Input: dimensioned drawing with shaded views. Units: mm. Origin: part minimum x, y, z. A direction names the side the tool comes from. Coordinates: 2 decimals unless noted, no trailing zeros. Write each loop counter-clockwise with the first axis right and the second up, starting at its lowest first coordinate (ties: lowest second). Pieces come first, ordered by that corner, then holes. Notation, with made-up numbers: M 85.5,-21 L 143.5,-21 A14 cw 143.5,-8 Z; hole C 82.25,12 d2. An arc over 180 degrees is marked long. Use one line per item in the form item = value.
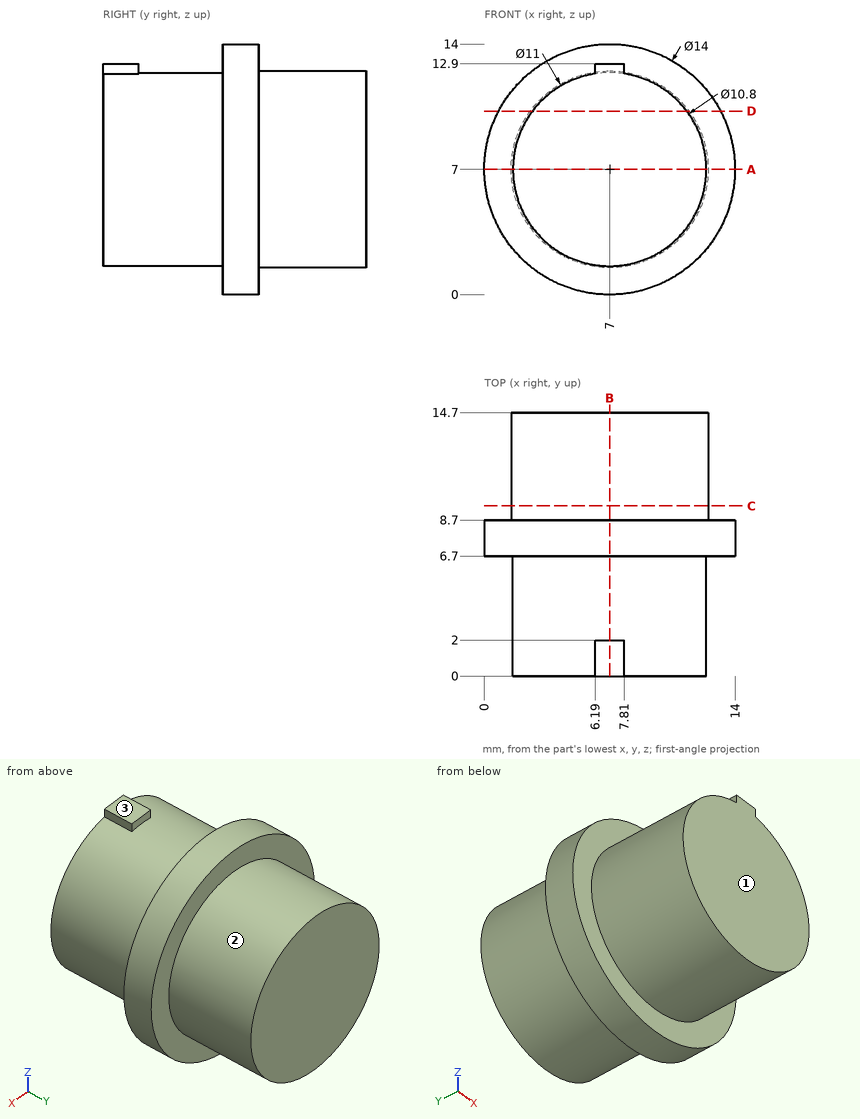
(1) Section query D-D on z = 10.25. Return the cut outline in (x, y).
Computed:
outline = M 0.8,6.7 L 2.69,6.7 L 2.69,0 L 11.31,0 L 11.31,6.7 L 13.2,6.7 L 13.2,8.7 L 11.44,8.7 L 11.44,14.7 L 2.56,14.7 L 2.56,8.7 L 0.8,8.7 Z
(2) Section query A-A on z = 7. Return the cut outline in (x, y), plus the area to 3 significant figures.
Computed:
outline = M 0,6.7 L 1.6,6.7 L 1.6,0 L 12.4,0 L 12.4,6.7 L 14,6.7 L 14,8.7 L 12.5,8.7 L 12.5,14.7 L 1.5,14.7 L 1.5,8.7 L 0,8.7 Z
area = 166 mm^2
(3) Section query C-C on y = 9.5. Return the cut outline in (x, z).
Computed:
outline = C 7,7 d11
(4) Set-up query: the marked faces 1, 2 and 3. Return all of +Z, -Z, +X, -X, +Y, -Y with unobstructed straight access to the full face (end or side cutting, diameter ignored); none if empty.
Computed:
face_1 = +Z, -Z, +X, -X, -Y
face_2 = +Y
face_3 = +Z, +X, -X, -Y
(5) First-contact query: pin 1 Ø2 at (x, z) = (3, 1.5) entering from +Y; pin 2 Ø1 at (y, z) = (6, 4.5) entering from +X; pin 3 Ø2 at (x, y) = (8, 5) entering from +Z. Flat tips, straight axial feed; report the tip coordinate or a pass-through.
Computed:
pin_1 = 8.7
pin_2 = 12.02
pin_3 = 12.4
(6) Section query B-B on x = 7. Return the cut outline in (y, z).
Computed:
outline = M 0,1.6 L 6.7,1.6 L 6.7,0 L 8.7,0 L 8.7,1.5 L 14.7,1.5 L 14.7,12.5 L 8.7,12.5 L 8.7,14 L 6.7,14 L 6.7,12.4 L 2,12.4 L 2,12.9 L 0,12.9 Z
(7) Line query: probe 1 along Y at (x, z) = (12.25, 5); probe 2 along X at (y, z) = (13.75, 2.5); probe 3 along X at (y, z) = (4.25, 4.75). Output: solid intervals per line, ascending.
Computed:
probe_1 = 6.7 to 8.7
probe_2 = 3.84 to 10.16
probe_3 = 2.09 to 11.91
